```python
from build123d import *

# Parameters (mm, degrees)
SKETCH_1_R      = 1.5
EXTRUDE_1_DEPTH = 4


with BuildPart() as part:
    # Эскиз1 → Бобышка-Вытянуть1 (new body)
    with BuildSketch(Plane.XY):
        with BuildLine():
            Line((4, 0), (4, 8.841521673))
            ThreePointArc((4, 8.841521673), (26.181376537, 11.5), (4, 14.158478327))
            Line((4, 14.158478327), (4, 23))
            Line((4, 23), (0, 23))
            Line((0, 23), (0, 0))
            Line((0, 0), (4, 0))
        make_face()
        with Locations((14.931376537, 11.5)):
            Circle(SKETCH_1_R, mode=Mode.SUBTRACT)
    extrude(amount=EXTRUDE_1_DEPTH)


solid = part.part
```
The model under review builds one solid part; all positions refer to its coordinate system, in mm. A direction names the side the tool comes from. Give positions to 0.01 mm unless a question says otherwise; leave off trailing zeros. Write each loop counter-clockwise with the first axis right and the second up, starting at its lowest first coordinate (ties: lowest second). Pieces come first, ordered by that corner, then holes. Notation, with made-up numbers: (-13.75, 5) -> (8.25, 5) arc R27 cw to (8.25, 30) -> close; hole circle Ø1 at (-37.5, -20). An arc over 180 degrees is marked (long way). Put each result on its own line as item: value.
(1) We need section D-D, the plane x = 21. Give the boundary of the cut face in (y, z), and give its area (3 significant figures).
Results are:
outline: (2.03, 0) -> (20.97, 0) -> (20.97, 4) -> (2.03, 4) -> close
area: 75.8 mm²
(2) To check wall thickness, follow probe 1 along X at (y, z) = (5.5, 2); probe 2 along X at (y, z) = (5.25, 1.05); probe 3 along Y at (x, z) = (15.5, 0.8). State the ranges of each line that lie inside material, in increasing order. Write a range as from..to.
Results are:
probe 1: 0..4, 5.41..24.45
probe 2: 0..4, 5.58..24.29
probe 3: 0.26..10.11, 12.89..22.74
(3) We need section C-C, the plane x = 15. Give the boundary of the cut face in (y, z).
Results are:
outline: (0.25, 0) -> (10, 0) -> (10, 4) -> (0.25, 4) -> close; (13, 0) -> (22.75, 0) -> (22.75, 4) -> (13, 4) -> close
(4) Tool access review of faces 1 (the flat face through (4, 4, 2)), 2 (the cylindrical face through (13.433, 11.566, 1.972)): name each direction out of +Z, -Z, +X, -X, +Y, -Y from which nothing blocks a thin tool from reaching the whole face with its end or side.
Results are:
face 1: +Z, -Z, -Y
face 2: +Z, -Z
(5) The part is to be moulded in two halves that separate along X. For faces 3 (the flat face through (0, 12, 2)), 4 (the flat face through (13, 12, 0)), 5 (the flat face through (4, 19, 2)), say which applies: pulls with the +X half, pulls with the -X half, needs draft (parallel to the pull), parting line crosses it, or undercut.
Results are:
face 3: pulls with the -X half
face 4: needs draft
face 5: undercut
(6) We need section A-A, the plane z = 2.85. Give the boundary of the cut face in (x, y), and give its area (3 significant figures).
Results are:
outline: (0, 0) -> (4, 0) -> (4, 8.84) arc R11.25 ccw (long way) to (4, 14.16) -> (4, 23) -> (0, 23) -> close; hole circle Ø3 at (14.93, 11.5)
area: 481 mm²
(7) We need section B-B, the plane y = 11.5. Give the boundary of the cut face in (x, z), and give its area (3 significant figures).
Results are:
outline: (0, 0) -> (13.43, 0) -> (13.43, 4) -> (0, 4) -> close; (16.43, 0) -> (26.18, 0) -> (26.18, 4) -> (16.43, 4) -> close
area: 92.7 mm²
(8) For pin 1 Ø4 at (x, y) = (14.93, 11.5) entering from -Z; pin 2 Ø1.2 at (y, z) = (19, 3) entering from +X; pin 3 Ø1 at (x, z) = (6.5, 1.5) entering from -Y; pin 4 Ø1.5 at (x, z) = (6, 1) entering from -Y, all flat-tipped, find the tip position at first contact; note any pin that passes through.
Results are:
pin 1: z = 0
pin 2: x = 23.82
pin 3: y = 3.52
pin 4: y = 3.78
